Geometry check sheet. Reference: the model listing, model coordinates, mm. A direction names the side the tool comes from. Give positions to 0.01 mm unless a question says otherwise; leave off trailing zeros. Loops run counter-clockwise (first coordinate to the right, second up) from the corner with the lowest first, then second, coordinate; pieces in that order, holes last. Notation, with made-up numbers: (84, 20.5) -> (107, 20.5) arc R12 cw to (107, 43.5) -> close; hole circle Ø1 at (-29.5, 52.5). An arc over 180 degrees is marked (long way). Answer as a JSON object with one key per item and string values.
from build123d import *

# Parameters (mm, degrees)
SKETCH1_W                = 25.5
SKETCH1_H                = 21.5
BOSS_EXTRUDE1_DEPTH      = 16
SKETCH3_W                = 30.5
SKETCH3_H                = 25.4
BOSS_EXTRUDE3_DEPTH      = 1.87
SKETCH4_W                = 23.8
SKETCH4_H                = 1
BOSS_EXTRUDE4_DEPTH      = 9.8
SKETCH5_W                = 0.8
SKETCH5_H                = 6.5
BOSS_EXTRUDE5_DEPTH      = 9.5
SKETCH6_W                = 8
SKETCH6_H                = 0.2
CUT_EXTRUDE1_DEPTH       = 28.15
CHAMFER1_SIZE            = 1
SKETCH7_R                = 1.5
CUT_EXTRUDE2_DEPTH       = 28.15
CHAMFER1_OF_MIRROR1_SIZE = 1
BOSS_EXTRUDE6_START      = -2
BOSS_EXTRUDE6_DEPTH      = 17.5
SKETCH9_W                = 24
SKETCH9_H                = 18.9
CUT_EXTRUDE3_DEPTH       = 5
SKETCH10_R               = 12.5
BOSS_EXTRUDE7_DEPTH      = 9.15
SKETCH11_R               = 40
CUT_EXTRUDE4_DEPTH       = 13.7
CUT_EXTRUDE4_DEPTH_BACK  = 13.7
CHAMFER2_SIZE            = 0.3


with BuildPart() as part:
    # Sketch1 → Boss-Extrude1 (new body)
    with BuildSketch(Plane.XY):
        Rectangle(SKETCH1_W, SKETCH1_H)
    extrude(amount=BOSS_EXTRUDE1_DEPTH)

    # Sketch3 → Boss-Extrude3 (add)
    with BuildSketch(Plane.XY.offset(16)):
        Rectangle(SKETCH3_W, SKETCH3_H)
    extrude(amount=BOSS_EXTRUDE3_DEPTH)

    # Sketch4 → Boss-Extrude4 (add)
    with BuildSketch(Plane(origin=(0, 0, 0), x_dir=(-1, 0, 0), z_dir=(0, 0, -1))):
        Rectangle(SKETCH4_W, SKETCH4_H)
    extrude(amount=BOSS_EXTRUDE4_DEPTH)

    # Sketch5 → Boss-Extrude5 (add)
    with BuildSketch(Plane(origin=(0, 0, 0), x_dir=(-1, 0, 0), z_dir=(0, 0, -1))):
        with Locations((11.5, -5.5)):
            Rectangle(SKETCH5_W, SKETCH5_H)
        with Locations((0, -5.5)):
            Rectangle(SKETCH5_W, SKETCH5_H)
        with Locations((-11.5, -5.5)):
            Rectangle(SKETCH5_W, SKETCH5_H)
    boss_extrude5 = extrude(amount=BOSS_EXTRUDE5_DEPTH)

    # Sketch6 → Cut-Extrude1 (cut, through all)
    with BuildSketch(Plane(origin=(11.9, 0, 0), x_dir=(0, 0, -1), z_dir=(1, 0, 0))):
        with Locations((5.5, -2.35)):
            Rectangle(SKETCH6_W, SKETCH6_H)
        with Locations((5.5, -8.65)):
            Rectangle(SKETCH6_W, SKETCH6_H)
    cut_extrude1 = extrude(amount=-CUT_EXTRUDE1_DEPTH, mode=Mode.SUBTRACT)

    # Chamfer1
    chamfer1_edges = [part.edges().sort_by_distance(p)[0] for p in [
        (-11.5, -2.45, -9.5),
        (0, -2.45, -9.5),
        (-11.5, -8.55, -9.5),
        (0, -8.55, -9.5),
        (11.5, -8.55, -9.5),
        (11.5, -2.45, -9.5),
    ]]
    chamfer(chamfer1_edges, length=CHAMFER1_SIZE)

    # Sketch7 → Cut-Extrude2 (cut, through all)
    with BuildSketch(Plane(origin=(11.9, 0, 0), x_dir=(0, 0, -1), z_dir=(1, 0, 0))):
        with Locations((6.5, -5.5)):
            Circle(SKETCH7_R)
        with Locations((2, -5.5)):
            Circle(SKETCH7_R)
    cut_extrude2 = extrude(amount=-CUT_EXTRUDE2_DEPTH, mode=Mode.SUBTRACT)

    # Mirror1: Boss-Extrude5, Cut-Extrude1, Cut-Extrude2 across plane
    add(boss_extrude5.mirror(Plane(origin=(0, 0, 0), x_dir=(0, 0, 1), z_dir=(0, -1, 0))))
    add(cut_extrude1.mirror(Plane(origin=(0, 0, 0), x_dir=(0, 0, 1), z_dir=(0, -1, 0))), mode=Mode.SUBTRACT)
    add(cut_extrude2.mirror(Plane(origin=(0, 0, 0), x_dir=(0, 0, 1), z_dir=(0, -1, 0))), mode=Mode.SUBTRACT)

    # Chamfer1 of Mirror1
    chamfer1_of_mirror1_edges = [part.edges().sort_by_distance(p)[0] for p in [
        (-11.5, 2.45, -9.5),
        (0, 2.45, -9.5),
        (-11.5, 8.55, -9.5),
        (0, 8.55, -9.5),
        (11.5, 8.55, -9.5),
        (11.5, 2.45, -9.5),
    ]]
    chamfer(chamfer1_of_mirror1_edges, length=CHAMFER1_OF_MIRROR1_SIZE)

    # Sketch8 → Boss-Extrude6 (add)
    with BuildSketch(Plane(origin=(0, 10.75, 0), x_dir=(1, 0, 0), z_dir=(0, 1, 0)).offset(BOSS_EXTRUDE6_START)):
        Polygon((-12.75, 0), (-14.15, -4.5), (-14.15, -12), (-13.754867215, -16), (-12.75, -16), (-13.15, -11.95072831), (-13.15, -4.651963334), (-12.75, -3.366249048), align=None)
    boss_extrude6 = extrude(amount=-BOSS_EXTRUDE6_DEPTH)

    # Mirror2: Boss-Extrude6 across plane
    add(boss_extrude6.mirror(Plane.ZY))

    # Sketch9 → Cut-Extrude3 (cut)
    with BuildSketch(Plane.XY.offset(17.87)):
        Rectangle(SKETCH9_W, SKETCH9_H)
    extrude(amount=-CUT_EXTRUDE3_DEPTH, mode=Mode.SUBTRACT)

    # Sketch10 → Boss-Extrude7 (add, symmetric)
    with BuildSketch(Plane(origin=(0, 0, 0), x_dir=(-1, 0, 0), z_dir=(0, -1, 0))):
        with Locations((0, -13.87)):
            Circle(SKETCH10_R)
    extrude(amount=BOSS_EXTRUDE7_DEPTH, both=True)

    # Sketch11 → Cut-Extrude4 (cut, two sides)
    with BuildSketch(Plane(origin=(0, 0, 0), x_dir=(-1, 0, 0), z_dir=(0, -1, 0))) as cut_extrude4_sk:
        with Locations((13, -58)):
            Circle(SKETCH11_R)
    extrude(amount=CUT_EXTRUDE4_DEPTH, mode=Mode.SUBTRACT)
    extrude(cut_extrude4_sk.sketch, amount=-CUT_EXTRUDE4_DEPTH_BACK, mode=Mode.SUBTRACT)

    # Chamfer2
    chamfer2_edges = [part.edges().sort_by_distance(p)[0] for p in [
        (-12, 0, 17.87),
        (0, 9.45, 17.87),
        (0, -9.45, 17.87),
        (12, 0, 17.87),
    ]]
    chamfer(chamfer2_edges, length=CHAMFER2_SIZE)


solid = part.part
1) Section check B-B on y = 5.5. Count the separate pieces of the cut face and the enclosed holes in it, plus the area to 3 significant figures.
Geometry check:
{"separate pieces": "7", "enclosed holes": "2", "area": "558 mm2"}
2) Material ranges on line 1 along Y through (x, z) = (-0.2, -6.5); line 2 along Y through (x, z) = (-11, 14); line 3 along X through (y, z) = (1.25, 7.5), recorded low to high. Write a range as from..to.
Geometry check:
{"line 1": "y = -8.55..-7, -4..-2.45, -0.5..0.5, 2.45..4, 7..8.55", "line 2": "y = -10.75..-9.45, -9.15..9.15, 9.45..10.75", "line 3": "x = -14.15..-13.15, -12.75..12.75, 13.15..14.15"}
3) Section check A-A on z = 11. Record the cut outline in (x, y).
Geometry check:
{"outline": "(-14.15, -8.75) -> (-13.15, -8.75) -> (-13.15, 8.75) -> (-14.15, 8.75) -> close; (-12.75, -10.75) -> (12.75, -10.75) -> (12.75, 10.75) -> (-12.75, 10.75) -> close; (13.15, -8.75) -> (14.15, -8.75) -> (14.15, 8.75) -> (13.15, 8.75) -> close"}
4) Section check C-C on x = 9. Record the cut outline in (y, z), plus the area to 3 significant figures.
Geometry check:
{"outline": "(-12.7, 16) -> (-10.75, 16) -> (-10.75, 0) -> (-0.5, 0) -> (-0.5, -9.8) -> (0.5, -9.8) -> (0.5, 0) -> (10.75, 0) -> (10.75, 16) -> (12.7, 16) -> (12.7, 17.87) -> (9.75, 17.87) -> (9.45, 17.57) -> (9.45, 12.87) -> (9.15, 12.87) -> (9.15, 22.54) -> (-9.15, 22.54) -> (-9.15, 12.87) -> (-9.45, 12.87) -> (-9.45, 17.57) -> (-9.75, 17.87) -> (-12.7, 17.87) -> close", "area": "484 mm2"}
5) Draft check along Z on faces 5 (the face through (-1.8, 0.1, 19.6)), 6 (the face through (-11.5, 8.55, -5)), 7 (the face through (0.01, -8.06, -8.99)), 8 (the face through (-13.955, 0.123, 13.972)). Enter one of: pulls with the +Z half, pulls with the -Z half, needs draft (parallel to the pull), parting line crosses it, or undercut.
Geometry check:
{"face 5": "pulls with the +Z half", "face 6": "needs draft", "face 7": "pulls with the -Z half", "face 8": "undercut"}
6) Depth check by flat-ended pin: P1, Ø0.9, axis at x = -11.5, z = -5.5, coming from the +Y side; P2, Ø3, axis at y = 4.5, z = -6, coming from the -X side; P3, Ø1.5, axis at y = 6.5, z = -5, coming from the +X side; P4, Ø2.5, axis at y = 5.5, z = -6.5, coming from the +X side. Enter the tip coordinate at first touch or a pass-through.
Geometry check:
{"P1": "stops at y = 8.55", "P2": "stops at x = -11.9", "P3": "stops at x = 11.9", "P4": "passes through"}
7) Tool access check on faces 1 (the face through (0, 8.75, -1)), 2 (the face through (3, -9.15, 17)), 3 (the face through (13.955, 0.123, 13.972)), 4 (the face through (-11.49, 2.96, -9.01)). Record the directions out of +Z, -Z, +X, -X, +Y, -Y that give a thin tool (end or side, any length) a straight path to the whole face; none if there is none.
Geometry check:
{"face 1": "-Z, +X, -X, +Y", "face 2": "+Z", "face 3": "+X, +Y, -Y", "face 4": "-Z, +X, -X"}
